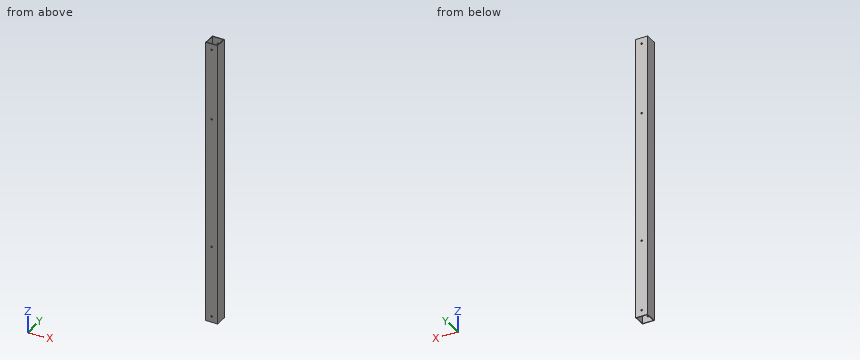
Autodesk Inventor part; units mm, degrees
ref_plane "YZ Plane" through (0, 0, 0) normal (1, 0, 0) x (0, 1, 0)
ref_plane "XZ Plane" through (0, 0, 0) normal (0, 1, 0) x (-1, 0, 0)
ref_plane "XY Plane" through (0, 0, 0) normal (0, 0, 1) x (1, 0, 0)
sketch "Sketch1" plane through (0, 0, 0) normal (0, 0, 1) x (1, 0, 0)
  line L0 (-14.0074, 10.2243) -> (11.3926, 10.2243)
  line L1 (11.3926, 10.2243) -> (11.3926, -15.1757)
  line L2 (11.3926, -15.1757) -> (-14.0074, -15.1757)
  line L3 (-14.0074, -15.1757) -> (-14.0074, 10.2243)
  line L4 (10.1226, 8.9543) -> (-12.7374, 8.9543)
  line L5 (-12.7374, 8.9543) -> (-12.7374, -13.9057)
  line L6 (-12.7374, -13.9057) -> (10.1226, -13.9057)
  line L7 (10.1226, -13.9057) -> (10.1226, 8.9543)
  point P0 (0, 0)
  dimension "d0" = 25.4
  dimension "d1" = 1.27
extrude "Extrusion2" add sketch "Sketch1" along normal blind 609.6
sketch "Sketch2" plane through (-14.0074, 10.2243, 0) normal (0, 1, 0) x (1, 0, 0)
  circle A0 centre (12.7, -165.1) radius 1.7272
  circle A1 centre (12.7, -444.5) radius 1.7272
  circle A2 centre (12.7, -596.9) radius 1.7272
  circle A3 centre (12.7, -12.7) radius 1.7272
  line L0 (12.7, -275.2188) -> (12.7, -289.6377) construction
  line L1 (25.4, -609.6) -> (0, -609.6)
  line L2 (25.4, 0) -> (25.4, -609.6)
  line L3 (25.4, 0) -> (0, 0)
  point P0 (14.0074, 0)
  dimension "d6" = 3.4544
  dimension "d7" = 12.7
  dimension "d8" = 12.7
  dimension "d9" = 12.7
  dimension "d11" = 152.4
  dimension "d15" = 152.4
extrude "Extrusion3" cut sketch "Sketch2" against normal through all
equation "\"d4\" = d2"
equation "\"d11\" = d14"
equation "\"d15\" = d14"
equation "\"d2\" = 609.6"
equation "\"d14\" = 152.4"
properties part number "24 in 1x1 for drive"
Can you work these out from the model? Positions are in its coordinate system, mm. Coordinates: 2 decimals unless noted, no trailing zeros. Order: outer loops, then holes, each group sorted by start corner. A loop starts at its lowest first (then second) coordinate and runs counter-clockwise, first axis right, second up. Notation, with made-up numbers: (43, 41) - (65, 41) arc R5 ccw to (65, 46) - close; hole circle Ø2 at (50, 17). An arc over 180 degrees is marked (long way). Answer as a JSON object with one key per item and string values. Group by question number.
Q1. Imagine slicing it at A-A (x = 6). Please give me the cut outline in (y, z), and give its area (3 significant figures).
Q2. Will these pins go through, and if not, where does the flat tip stop? P1, Ø3, axis at x = -1.31, z = 444.5, coming from the -Y side; P2, Ø4, axis at x = -1.31, z = 596.9, coming from the +Y side.
Q3. I need wall thicknesses on line 1 (X direction, y = 9.75, z = 12.7); line 2 (X direction, y = 2.25, z = 554); line 3 (Y direction, x = -2.5, z = 202.5). Which ranges of each line are inside material? Lowest first, please. Write a range as from..to.
Q4. Imagine slicing it at C-C (y = -2.5). Please give me the cut outline in (x, z).
Q5. Imagine slicing it at B-B (z = 354.5). Please give me the cut outline in (x, y).
Determined:
{
 "1": {"outline": "(-15.18, 0) - (-13.91, 0) - (-13.91, 609.6) - (-15.18, 609.6) - close; (8.95, 0) - (10.22, 0) - (10.22, 609.6) - (8.95, 609.6) - close", "area": "1,550 mm2"},
 "2": {"P1": "passes through", "P2": "stops at y = 10.22"},
 "3": {"line 1": "x = -14.01..-3.03, 0.42..11.39", "line 2": "x = -14.01..-12.74, 10.12..11.39", "line 3": "y = -15.18..-13.91, 8.95..10.22"},
 "4": {"outline": "(-14.01, 0) - (-12.74, 0) - (-12.74, 609.6) - (-14.01, 609.6) - close; (10.12, 0) - (11.39, 0) - (11.39, 609.6) - (10.12, 609.6) - close"},
 "5": {"outline": "(-14.01, -15.18) - (11.39, -15.18) - (11.39, 10.22) - (-14.01, 10.22) - close; hole (-12.74, -13.91) - (10.12, -13.91) - (10.12, 8.95) - (-12.74, 8.95) - close"}
}
